from build123d import *

# Parameters (mm, degrees)
RESSALTO_EXTRUS_O1_DEPTH = 40
CASCA1_T                 = 0.5
ESBO_O2_W                = 31
ESBO_O2_H                = 20
RESSALTO_EXTRUS_O2_DEPTH = 3
FILETE1_R                = 20
FILETE2_R                = 20
ESBO_O3_R                = 2
CORTE_EXTRUS_O1_DEPTH    = 106.198621664
FILETE3_R                = 1
FILETE4_R                = 1


with BuildPart() as part:
    # Esboço1 → Ressalto-extrusão1 (new body)
    with BuildSketch(Plane.XY):
        Polygon((-16.000735804, -69), (-16.000735804, -49), (15.999264196, -49), (15.999264196, -69), (28.580735804, -69), (69, -28.580735804), (69, -15.500735804), (47, -15.500735804), (47, 16.499264196), (69, 16.499264196), (69, 28.580735804), (28.580735804, 69), (15.999264196, 69), (15.999264196, 49), (-16.000735804, 49), (-16.000735804, 69), (-28.580735804, 69), (-69, 28.580735804), (-69, 16.499264196), (-47, 16.499264196), (-47, -15.500735804), (-69, -15.500735804), (-69, -28.580735804), (-28.580735804, -69), align=None)
    extrude(amount=RESSALTO_EXTRUS_O1_DEPTH)

    # Casca1
    casca1_openings = [part.faces().sort_by_distance(p)[0] for p in [
        (7.1958e-05, -0.05370825, 0),
    ]]
    offset(amount=CASCA1_T, openings=casca1_openings, kind=Kind.INTERSECTION)

    # Esboço2 → Ressalto-extrusão2 (add)
    with BuildSketch(Plane.XY):
        with Locations((-0.000735804, -59.5)):
            Rectangle(ESBO_O2_W, ESBO_O2_H)
        with Locations((-0.000735804, 59.5)):
            Rectangle(ESBO_O2_W, ESBO_O2_H)
    extrude(amount=RESSALTO_EXTRUS_O2_DEPTH)

    # Filete1
    filete1_edges = [part.edges().sort_by_distance(p)[0] for p in [
        (-49.143921292, 49.143921292, 40.5),
        (49.143921292, -49.143921292, 40.5),
        (-49.143921292, -49.143921292, 40.5),
        (49.143921292, 49.143921292, 40.5),
    ]]
    fillet(filete1_edges, radius=FILETE1_R)

    # Filete2
    filete2_edges = [part.edges().sort_by_distance(p)[0] for p in [
        (-48.790367902, 48.790367902, 40),
        (-48.790367902, -48.790367902, 40),
        (48.790367902, -48.790367902, 40),
        (48.790367902, 48.790367902, 40),
    ]]
    fillet(filete2_edges, radius=FILETE2_R)

    # Esboço3 → Corte-extrusão1 (cut, through all)
    with BuildSketch(Plane.XY.offset(3)):
        with Locations((-10.500735804, -54.5)):
            Circle(ESBO_O3_R)
        with Locations((-10.500735804, -64.5)):
            Circle(ESBO_O3_R)
        with Locations((10.439264196, -64.5)):
            Circle(ESBO_O3_R)
        with Locations((10.439264196, -54.5)):
            Circle(ESBO_O3_R)
        with Locations(Location((10.439264196, 54.5, 0), (0, 0, 180))):
            Circle(ESBO_O3_R)
        with Locations(Location((10.439264196, 64.5, 0), (0, 0, 180))):
            Circle(ESBO_O3_R)
        with Locations(Location((-10.500735804, 64.5, 0), (0, 0, 180))):
            Circle(ESBO_O3_R)
        with Locations(Location((-10.500735804, 54.5, 0), (0, 0, 180))):
            Circle(ESBO_O3_R)
    extrude(amount=-CORTE_EXTRUS_O1_DEPTH, mode=Mode.SUBTRACT)

    # Filete3
    # the kernel refuses this fillet: 1 mm, written as the material it takes off along each edge
    with BuildSketch(Plane(origin=(31.287842585, -69.5, 0), x_dir=(0, 1, 0), z_dir=(-1, 0, 0))) as filete3_piece_1:
        with BuildLine():
            CenterArc((FILETE3_R, -FILETE3_R), FILETE3_R, 90, 90)
            Line((0, -FILETE3_R), (0, 0))
            Line((0, 0), (FILETE3_R, 0))
        make_face()
    extrude(amount=62.57568517, mode=Mode.SUBTRACT)

    # Filete4
    # the kernel refuses this fillet: 1 mm, written as the material it takes off along each edge
    with BuildSketch(Plane(origin=(-31.287842585, 69.5, 0), x_dir=(0, -1, 0), z_dir=(1, 0, 0))) as filete4_piece_1:
        with BuildLine():
            CenterArc((FILETE4_R, -FILETE4_R), FILETE4_R, 90, 90)
            Line((0, -FILETE4_R), (0, 0))
            Line((0, 0), (FILETE4_R, 0))
        make_face()
    extrude(amount=62.57568517, mode=Mode.SUBTRACT)


solid = part.part
Can you work these out from the model? Positions are in its coordinate system, mm. A direction names the side the tool comes from. Coordinates: 2 decimals unless noted, no trailing zeros. Loops run counter-clockwise (first coordinate to the right, second up) from the corner with the lowest first, then second, coordinate; pieces in that order, holes last. Notation, with made-up numbers: M -32.5,15 L -10.5,15 A13 cw -10.5,34 Z; hole C 66.25,-8 d8. An arc over 180 degrees is marked long. Return JSON: item names as keys, results as strings. Group by question number.
Item 1: Imagine slicing it at A-A (x = -1). Please give me the cut outline in (y, z).
Item 2: Imagine slicing it at B-B (y = 3). Please give me the cut outline in (x, z), and give its area (3 significant figures).
Item 3: Imagine slicing it at C-C (y = 64.5). Give the number of separate pieces and of enclosed holes in the cut face, and give its area (3 significant figures).
Item 4: On a 3-axis mill with a long thin cutter (end or side, diameter ignored), from which of +Z, -Z, +X, -X, +Y, -Y can I reach the whole of each face in a straight line? I mean faces 1 (the flat face through (-15.501, 59, 21)), 2 (the flat face through (22, 69, 18)), 3 (the flat face through (-58, -15.001, 20)), 4 (the flat face through (0, -49.5, 21)), 5 (the flat face through (59, -15.001, 20)). Say none if no direction works.
Item 5: Thinking about a two-plate mould opening in X: for faces 6 (the flat face through (69.5, 22, 18)), 7 (the flat face through (-0.4, -69.5, 2.8)), 8 (the flat face through (15.499, 60, 21)), which applies, released by +X, released by -X, zero draft, split by the parting line, or undercut?
Item 6: I'm going to push flat-ended pins straight in: pin 1 Ø11 at (x, z) = (54, 18) entering from +Y; pin 2 Ø24 at (x, z) = (-56.5, 20.5) entering from +Y; pin 3 Ø12 at (x, z) = (-51.5, 5.5) entering from -Y. Where does each tip first touch, or does it pass through?
Item 7: If I drill on L1, parallel to Y at x = -10, z = 4.5; L2, parallel to Y at x = 28, z = 4; L3, parallel to Y at x = 60, z = 25.5, over which ranges is the centre line in solid material (lowest first)? Write a range as from..to.
Verdict:
{
 "1": {"outline": "M -69.5,1 A1 ccw -68.5,0 L -49,0 L -49,40 L 49,40 L 49,0 L 68.5,0 A1 ccw 69.5,1 L 69.5,3 L 49.5,3 L 49.5,40.5 L -49.5,40.5 L -49.5,3 L -69.5,3 Z"},
 "2": {"outline": "M -47.5,0 L -47,0 L -47,40 L 47,40 L 47,0 L 47.5,0 L 47.5,40.5 L -47.5,40.5 Z", "area": "87.5 mm^2"},
 "3": {"separate pieces": "3", "enclosed holes": "0", "area": "180 mm^2"},
 "4": {"face 1": "+Z, +Y", "face 2": "-Z", "face 3": "+Z, -Z, -X", "face 4": "+Z, -Y", "face 5": "+Z, -Z, +X"},
 "5": {"face 6": "released by +X", "face 7": "zero draft", "face 8": "undercut"},
 "6": {"pin 1": "stops at y = 49.79", "pin 2": "stops at y = 53.79", "pin 3": "stops at y = -52.79"},
 "7": {"L1": "y = -49.5..-49, 49..49.5", "L2": "y = -69.5..-69, 69..69.5", "L3": "y = -37.39..-36.49, -15.5..-15, 16..16.5, 36.49..37.39"}
}
